For this review, take the finished solid that the model builds, in its own axes (mm). Give positions to 0.01 mm unless a question says otherwise; leave off trailing zeros. Loops run counter-clockwise (first coordinate to the right, second up) from the corner with the lowest first, then second, coordinate; pieces in that order, holes last. Notation, with made-up numbers: (80, -18) -> (104, -18) arc R19 ccw to (104, -7) -> close; hole circle Ø1 at (31, 44.5). An arc over 180 degrees is marked (long way). Answer as CSV lines item,"result". Start each with the question number.
Item 1: Add section B-B on y = -4. State the section outline as (x, z) points, plus the area to 3 significant figures.
Item 2: Add section C-C on x = -67.5. State the section outline as (y, z) points.
Item 3: Add section D-D on z = -0.85. State how many separate pieces and enclosed holes the cut face has, plus the area to 3 significant figures.
Item 4: Add section A-A on x = 13.5. State the section outline as (y, z) points.
Item 5: For L1, parallel to X at y = -9.5, z = 1.6; L2, parallel to Y at x = 51.5, z = -0.65 (3 decimals); L3, parallel to X at y = 18.5, z = -0.2, list the stretches that pass through material, from the lowest coordinate up. Write a range as from..to.
Item 6: Clearance check with flat-ended pins moving along their axes: P1, Ø1.2, axis at x = -79.5, z = 0, coming from the -Y side; P2, Ø2, axis at x = -71, z = -0.5, coming from the -Y side. State where each tip first meets the part, or that it passes through.
```python
from build123d import *

# Parameters (mm, degrees)
SKETCH_1_W          = 176
SKETCH_1_H          = 50
EXTRUDE_1_DEPTH     = 2
SKETCH_2_R          = 2.025
CUT_EXTRUDE_1_DEPTH = 22
CUT_EXTRUDE_2_DEPTH = 17
FILLET_1_R          = 2
SKETCH_4_R          = 2.025
CUT_EXTRUDE_3_DEPTH = 5
CUT_EXTRUDE_5_DEPTH = 15.5
SKETCH_8_W          = 22.857142857
SKETCH_8_H          = 30
CUT_EXTRUDE_6_DEPTH = 15.5
FILLET_2_R          = 2
SKETCH_11_W         = 42
SKETCH_11_H         = 10
EXTRUDE_4_DEPTH     = 4
SKETCH_12_R         = 1.51
CUT_EXTRUDE_8_DEPTH = 4
SKETCH_13_R         = 1.5
CUT_EXTRUDE_9_DEPTH = 10
EXTRUDE_5_DEPTH     = 4
FILLET_3_R          = 2
FILLET_4_R          = 2


with BuildPart() as part:
    # 草图1 → 凸台-拉伸1 (new, symmetric)
    with BuildSketch(Plane.XY):
        Rectangle(SKETCH_1_W, SKETCH_1_H)
    extrude(amount=EXTRUDE_1_DEPTH, both=True)

    # 草图2 → 切除-拉伸1 (cut, symmetric)
    with BuildSketch(Plane(origin=(0, 0, -2), x_dir=(-1, 0, 0), z_dir=(0, 0, -1))):
        with Locations((51.5, 21)):
            Circle(SKETCH_2_R)
        with Locations((51.5, -21)):
            Circle(SKETCH_2_R)
        with Locations((83.5, 21)):
            Circle(SKETCH_2_R)
        with Locations((83.5, -21)):
            Circle(SKETCH_2_R)
    cut_extrude_1 = extrude(amount=CUT_EXTRUDE_1_DEPTH, both=True, mode=Mode.SUBTRACT)

    # 镜向1: 切除-拉伸1 across plane
    add(cut_extrude_1.mirror(Plane(origin=(0, 0, 0), x_dir=(0, 0, 1), z_dir=(1, 0, 0))), mode=Mode.SUBTRACT)

    # 草图3 → 切除-拉伸2 (cut, symmetric)
    with BuildSketch(Plane(origin=(0, 0, -2), x_dir=(-1, 0, 0), z_dir=(0, 0, -1))):
        with BuildLine():
            Line((63.5, -21), (63.5, -25))
            Line((63.5, -25), (71.5, -25))
            Line((71.5, -25), (71.5, -21))
            ThreePointArc((71.5, -21), (67.5, -17), (63.5, -21))
        make_face()
    cut_extrude_2 = extrude(amount=CUT_EXTRUDE_2_DEPTH, both=True, mode=Mode.SUBTRACT)

    # 镜向2: 切除-拉伸2 across plane
    add(cut_extrude_2.mirror(Plane(origin=(0, 0, 0), x_dir=(0, 0, 1), z_dir=(1, 0, 0))), mode=Mode.SUBTRACT)

    # 圆角1
    fillet_1_edges = [part.edges().sort_by_distance(p)[0] for p in [
        (-71.5, -25, 0),
        (-63.5, -25, 0),
        (88, -25, 0),
        (-88, -25, 0),
        (-88, 25, 0),
        (88, 25, 0),
        (63.5, -25, 0),
        (71.5, -25, 0),
    ]]
    fillet(fillet_1_edges, radius=FILLET_1_R)

    # 草图4 → 切除-拉伸3 (cut, symmetric)
    with BuildSketch(Plane(origin=(0, 0, -2), x_dir=(-1, 0, 0), z_dir=(0, 0, -1))):
        with Locations((47.5, -12.5)):
            Circle(SKETCH_4_R)
        with Locations((47.5, 12.5)):
            Circle(SKETCH_4_R)
        with Locations((-47.5, 12.5)):
            Circle(SKETCH_4_R)
        with Locations((-47.5, -12.5)):
            Circle(SKETCH_4_R)
    extrude(amount=CUT_EXTRUDE_3_DEPTH, both=True, mode=Mode.SUBTRACT)

    # 草图7 → 切除-拉伸5 (cut, symmetric)
    with BuildSketch(Plane.XY.offset(2)):
        Polygon((-2, 19), (-45.032854639, 19), (-43.5, 15.742683893), (-43.5, -15.742683893), (-45.032854639, -19), (-2, -19), align=None)
        Polygon((45.032854639, 19), (2, 19), (2, -19), (45.032854639, -19), (43.5, -15.742683893), (43.5, 15.742683893), align=None)
    extrude(amount=CUT_EXTRUDE_5_DEPTH, both=True, mode=Mode.SUBTRACT)

    # 草图8 → 切除-拉伸6 (cut, symmetric)
    with BuildSketch(Plane.XY.offset(2)):
        with Locations((-69.023809524, 2)):
            Rectangle(SKETCH_8_W, SKETCH_8_H)
        with Locations((69.023809524, 2)):
            Rectangle(SKETCH_8_W, SKETCH_8_H)
    extrude(amount=CUT_EXTRUDE_6_DEPTH, both=True, mode=Mode.SUBTRACT)

    # 圆角2
    fillet_2_edges = [part.edges().sort_by_distance(p)[0] for p in [
        (-2, 19, 0),
        (-2, -19, 0),
        (-45.032854639, -19, 0),
        (-43.5, -15.742683893, 0),
        (-43.5, 15.742683893, 0),
        (-45.032854639, 19, 0),
        (2, 19, 0),
        (45.032854639, 19, 0),
        (43.5, 15.742683893, 0),
        (43.5, -15.742683893, 0),
        (45.032854639, -19, 0),
        (2, -19, 0),
        (-80.452380952, -13, 0),
        (-80.452380952, 17, 0),
        (-57.595238095, 17, 0),
        (-57.595238095, -13, 0),
        (80.452380952, 17, 0),
        (80.452380952, -13, 0),
        (57.595238095, -13, 0),
        (57.595238095, 17, 0),
    ]]
    fillet(fillet_2_edges, radius=FILLET_2_R)

    # 草图11 → 凸台-拉伸4 (add)
    with BuildSketch(Plane.XY.offset(2)):
        with Locations((-9, -30)):
            Rectangle(SKETCH_11_W, SKETCH_11_H)
    extrude(amount=-EXTRUDE_4_DEPTH)

    # 草图12 → 切除-拉伸8 (cut)
    with BuildSketch(Plane.XY.offset(2)):
        with Locations((-4, -32)):
            Circle(SKETCH_12_R)
        with Locations((-24, -32)):
            Circle(SKETCH_12_R)
    extrude(amount=-CUT_EXTRUDE_8_DEPTH, mode=Mode.SUBTRACT)

    # 草图13 → 切除-拉伸9 (cut)
    with BuildSketch(Plane.XY.offset(2)):
        with Locations((-31.5, -25)):
            Circle(SKETCH_13_R)
        with Locations((13.5, -25)):
            Circle(SKETCH_13_R)
    extrude(amount=-CUT_EXTRUDE_9_DEPTH, mode=Mode.SUBTRACT)

    # 草图14 → 凸台-拉伸5 (add)
    with BuildSketch(Plane.XY.offset(2)):
        with BuildLine():
            Line((-2, -15), (-43.5, -15))
            Line((-43.5, -15), (-43.5, -15.295610336))
            ThreePointArc((-43.5, -15.295610336), (-43.548170754, -15.731915957), (-43.690362596, -16.147204408))
            Line((-43.690362596, -16.147204408), (-43.690928016, -16.148405927))
            ThreePointArc((-43.690928016, -16.148405927), (-43.569956971, -18.071637032), (-41.881290612, -19))
            Line((-41.881290612, -19), (-4, -19))
            ThreePointArc((-4, -19), (-2.585786438, -18.414213562), (-2, -17))
            Line((-2, -17), (-2, -15))
        make_face()
        with BuildLine():
            Line((43.5, -15), (2, -15))
            Line((2, -15), (2, -17))
            ThreePointArc((2, -17), (2.585786438, -18.414213562), (4, -19))
            Line((4, -19), (41.881290612, -19))
            ThreePointArc((41.881290612, -19), (43.569956971, -18.071637032), (43.690928016, -16.148405927))
            Line((43.690928016, -16.148405927), (43.690362596, -16.147204408))
            ThreePointArc((43.690362596, -16.147204408), (43.548170754, -15.731915957), (43.5, -15.295610336))
            Line((43.5, -15.295610336), (43.5, -15))
        make_face()
    extrude(amount=-EXTRUDE_5_DEPTH)

    # 圆角3
    fillet_3_edges = [part.edges().sort_by_distance(p)[0] for p in [
        (-2, -15, 0),
        (-43.5, -15, 0),
        (43.5, -15, 0),
        (2, -15, 0),
    ]]
    fillet(fillet_3_edges, radius=FILLET_3_R)

    # 圆角4
    fillet_4_edges = [part.edges().sort_by_distance(p)[0] for p in [
        (12, -35, 0),
        (-30, -35, 0),
    ]]
    fillet(fillet_4_edges, radius=FILLET_4_R)


solid = part.part
```
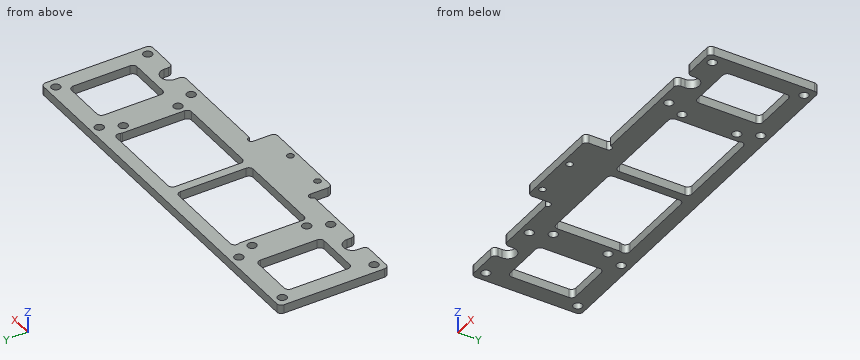
Computed values:
1,outline,"(-88, -2) -> (-80.45, -2) -> (-80.45, 2) -> (-88, 2) -> close; (-57.6, -2) -> (-43.5, -2) -> (-43.5, 2) -> (-57.6, 2) -> close; (-2, -2) -> (2, -2) -> (2, 2) -> (-2, 2) -> close; (43.5, -2) -> (57.6, -2) -> (57.6, 2) -> (43.5, 2) -> close; (80.45, -2) -> (88, -2) -> (88, 2) -> (80.45, 2) -> close"
1,area,"189 mm²"
2,outline,"(-17, -2) -> (-13, -2) -> (-13, 2) -> (-17, 2) -> close; (17, -2) -> (25, -2) -> (25, 2) -> (17, 2) -> close"
3,separate pieces,"1"
3,enclosed holes,"18"
3,area,"4,740 mm²"
4,outline,"(-23.5, -2) -> (-15, -2) -> (-15, 2) -> (-23.5, 2) -> close; (19, -2) -> (25, -2) -> (25, 2) -> (19, 2) -> close"
5,L1,"-88..-80.45, -57.6..-43.5, -2..2, 43.5..57.6, 80.45..88"
5,L2,"-25..-23.025, -18.975..18.975, 23.025..25"
5,L3,"-88..-43.2, -2.68..2.68, 43.2..88"
6,P1,"y = -25"
6,P2,"y = -24.32"
